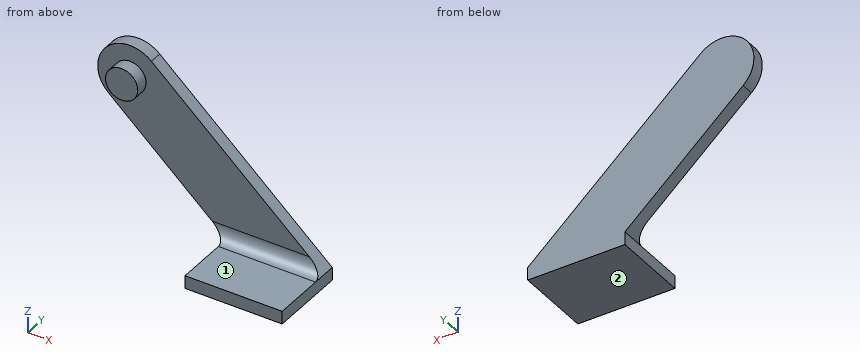
```python
from build123d import *

# Parameters (mm, degrees)
F0_R          = 2.5
F1_DEPTH      = 2
F0_W          = 15.064
F0_H          = 2
F2_DEPTH      = 10
F2_DEPTH_BACK = 2
F3_DEPTH      = 2
F3_DEPTH_BACK = 2
F4_R          = 2


# Not quite as in the source:
# - ends of sketch curves that miss each other by under 0.0002 mm in the source are joined


with BuildPart() as f1:
    # F0 (on Front) → F1 (new body)
    with BuildSketch(Plane.XZ):
        with BuildLine():
            Line((30.0639452948, -20), (3.3191835885, 3.7393876913))
            ThreePointArc((3.3191835885, 3.7393876913), (-3.7393876913, 3.3191835885), (-3.3191835885, -3.7393876913))
            Line((-3.3191835885, -3.7393876913), (15, -20))
            Line((15, -20), (30.0639452948, -20))
        make_face()
        Circle(F0_R, mode=Mode.SUBTRACT)
    extrude(amount=-F1_DEPTH)

    # F0 (on Front) → F2 (join, two sides)
    with BuildSketch(Plane.XZ) as f2_sk:
        with Locations((22.532, -21)):
            Rectangle(F0_W, F0_H)
    extrude(amount=F2_DEPTH)
    extrude(f2_sk.sketch, amount=-F2_DEPTH_BACK)

    # F0 (on Front) → F3 (join, two sides)
    with BuildSketch(Plane.XZ) as f3_sk:
        Circle(F0_R)
    extrude(amount=F3_DEPTH)
    extrude(f3_sk.sketch, amount=-F3_DEPTH_BACK)

    # F4
    f4_edges = [f1.edges().sort_by_distance(p)[0] for p in [
        (22.531973, 0, -20),
    ]]
    fillet(f4_edges, radius=F4_R)


solid = f1.part
```
The listing builds one solid part. Answer for the finished solid, in the listing's coordinates (mm). Face numbers are marked on the shaded views. A direction names the side the tool comes from. Give positions to 0.01 mm unless a question says otherwise; leave off trailing zeros. Order: outer loops, then holes, each group sorted by start corner. A loop starts at its lowest first (then second) coordinate and runs counter-clockwise, first axis right, second up. Notation, with made-up numbers: (66, -35) -> (82, -35) arc R21 ccw to (82, -29) -> close; hole circle Ø8 at (-12, -36). An arc over 180 degrees is marked (long way). Answer as CSV lines item,"result". Start each with the question number.
Q1. A cutting plane is placed at B-B (x = 16). Determine the outline of the cut face in (y, z).
Q2. A cutting plane is placed at D-D (x = 0). Determine the outline of the cut face in (y, z), then the cut area to 3 significant figures.
Q3. Which of the six approach directions +Z, -Z, +X, -X, +Y, -Y give full straight-line access (tool end or side, diameter ignored) to the marked faces 1 and 2?
Q4. Given pin 1 (0.6 mm diameter, centred on y = -5, z = -20.5, fed in from -X); pin 2 (2.5 mm diameter, centred on x = -1, z = 0.5, fed in from -Y); pin 3 (4 mm diameter, centred on y = -6.5, z = -16.5, fed in from +X); pin 4 (11.5 mm diameter, centred on x = 16.5, z = -4.5, fed in from -Y), each flat-ended and moving along its own axis, determine where each tip first touches the part or whether it passes through.
Q5. Find the intervals of material crossed by L1, parallel to Y at x = 14, z = -16.25; L2, parallel to Z at x = 16, y = -6; L3, parallel to Z at x = 8, y = 1, in increasing order.
Q6. A cutting plane is placed at A-A (z = 0). Determine the outline of the cut face in (x, y).
Results found:
1,outline,"(-10, -22) -> (2, -22) -> (2, -7.52) -> (0, -7.52) -> (0, -18) arc R2 cw to (-2, -20) -> (-10, -20) -> close"
2,outline,"(-2, -2.5) -> (0, -2.5) -> (0, -6.69) -> (2, -6.69) -> (2, 5) -> (0, 5) -> (0, 2.5) -> (-2, 2.5) -> close"
2,area,"33.4 mm2"
3,face 1,"+Z, +X, -X, -Y"
3,face 2,"-Z, +X, -X, +Y, -Y"
4,pin 1,"x = 15"
4,pin 2,"y = -2"
4,pin 3,"through"
4,pin 4,"y = 0"
5,L1,"0 to 2"
5,L2,"-22 to -20"
5,L3,"-13.79 to -0.42"
6,outline,"(-5, 0) -> (-2.5, 0) -> (-2.5, -2) -> (2.5, -2) -> (2.5, 0) -> (7.53, 0) -> (7.53, 2) -> (-5, 2) -> close"
